For this review, use the dimensioned drawing (mm, ordinates from the lowest corner) and the shaded views. Round coordinates to 2 decimals unless told otherwise and drop trailing zeros. Write each loop counter-clockwise with the first axis right and the second up, starting at its lowest first coordinate (ties: lowest second). Pieces come first, ordered by that corner, then holes. Notation, with made-up numbers: (9, 17) - (51, 17) arc R21 cw to (51, 26) - close; hole circle Ø4 at (-9.5, 69.5). An arc over 180 degrees is marked (long way). Return JSON: item names as keys, results as strings.
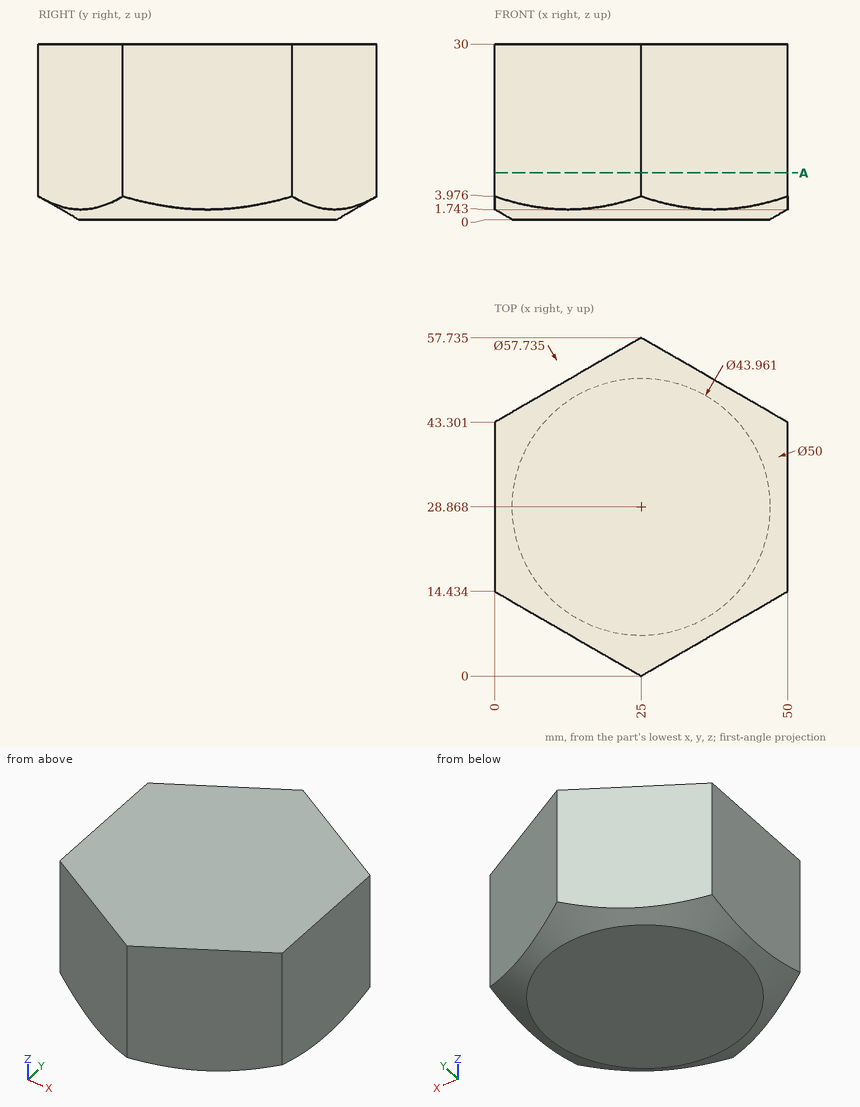
(1) Wall thickness on line 1 (X direction, y = 44, z = 26); line 2 (X direction, y = 55.5, z = 17.25) (1 decimal); line 3 (Y direction, x = 6, z = 14) (1 decimal): over which ranges is each line inside the solid? List them lowest first.
Filled in:
{"line 1": "x = 1.21 to 48.79", "line 2": "x = 21.1 to 28.9", "line 3": "y = 11 to 46.8"}
(2) Add section A-A (z = 8). Write out the cut boundary in (x, y) (1 decimal), plus the area to 4 significant figures.
Filled in:
{"outline": "(0, 14.4) - (25, 0) - (50, 14.4) - (50, 43.3) - (25, 57.7) - (0, 43.3) - close", "area": "2,165 mm2"}
(3) Clearance check with flat-ended pins moving along their axes: pin 1 Ø1 at (x, z) = (38.5, 12.5) entering from +Y; pin 2 Ø1.5 at (x, y) = (42.5, 11) entering from -Z (1 decimal); pin 3 Ø10 at (x, y) = (42.5, 15) entering from -Z; pin 4 Ø6 at (x, z) = (35.5, 24.5) entering from +Y (1 decimal). State where each tip first meets the part, or that it passes through.
Filled in:
{"pin 1": "stops at y = 50.23", "pin 2": "stops at z = 1.3", "pin 3": "stops at z = 0", "pin 4": "stops at y = 53.4"}
